Source: three-view drawing plus pictorial views. Frame: mm from the lowest corner of the part. A direction names the side the tool comes from. Give positions to 0.01 mm unless a question says otherwise; leave off trailing zeros. Order: outer loops, then holes, each group sorted by start corner. A loop starts at its lowest first (then second) coordinate and runs counter-clockwise, first axis right, second up. Notation, with made-up numbers: M 3,77 L 47,77 A9 cw 47,83 Z; hole C -15.5,47.25 d5. An arc over 180 degrees is marked long. Use CSV: the item, a comma, the result in double quotes.
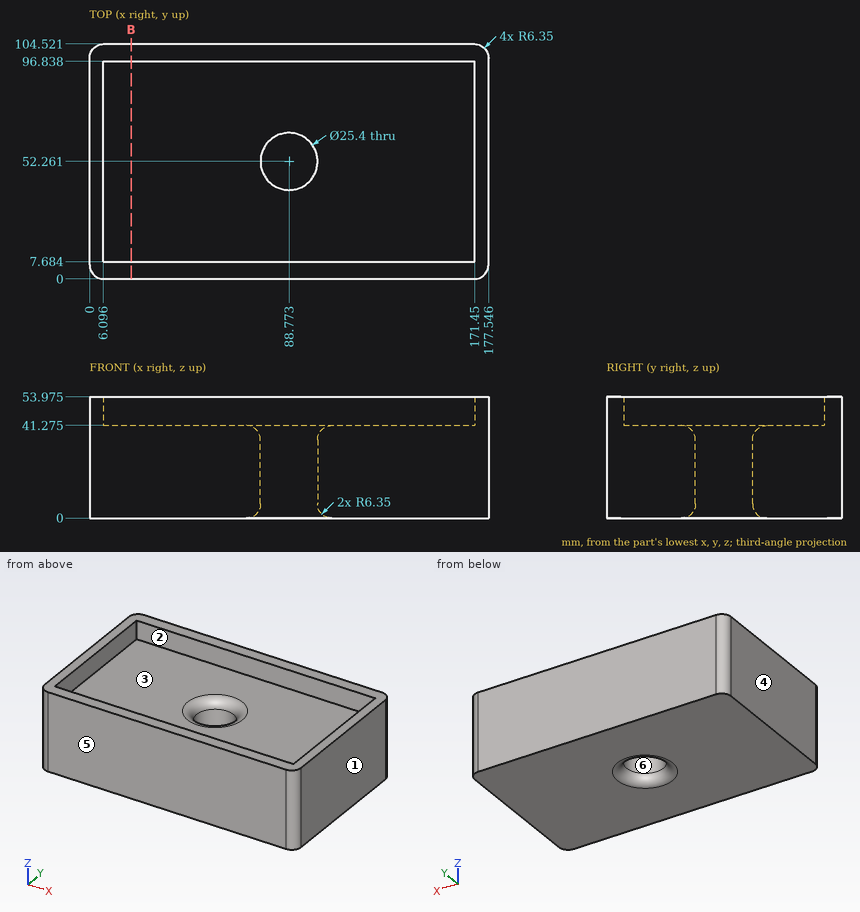
1. Pull-direction query (X, two-part tool) for the marked faces 3, 4, 5 and 6; classes: +X half, -X half, draft (parallel to the pull), parting line (faces both ways), or undercut.
Answer:
face 3,"undercut"
face 4,"-X half"
face 5,"draft"
face 6,"undercut"
2. Line query: line 1 (Y direction, x = 127.5, z = 46); line 2 (Z direction, x = 118, y = 91.5) (1 decimal); line 3 (Y direction, x = 83, z = 4.5). Output: solid intervals per line, ascending.
Answer:
line 1,"0 to 7.68, 96.84 to 104.52"
line 2,"0 to 41.3"
line 3,"0 to 40.64, 63.88 to 104.52"
3. Pin query (flat end, axial travel): pin 1 Ø1 at (x, y) = (73.5, 46.5) entering from -Z. Return the tip coordinate at first contact, or that it passes through.
Answer:
pin 1,"z = 0.4"
4. Section B-B, the plane x = 18.5. Return the cut outline in (y, z) (1 decimal), plus the area to 3 significant figures.
Answer:
outline,"M 0,0 L 104.5,0 L 104.5,54 L 96.8,54 L 96.8,41.3 L 7.7,41.3 L 7.7,54 L 0,54 Z"
area,"4,510 mm2"
5. Reachability of the marked faces 1 and 2 from +Z, -Z, +X, -X, +Y, -Y: full face, straight path, thin tool, end or side. Return the list, or none.
Answer:
face 1,"+Z, -Z, +X, +Y, -Y"
face 2,"+Z"
